Part model, mm, in its own coordinate system. A direction names the side the tool comes from. Round coordinates to 2 decimals unless told otherwise and drop trailing zeros. Write each loop counter-clockwise with the first axis right and the second up, starting at its lowest first coordinate (ties: lowest second). Pieces come first, ordered by that corner, then holes. Notation, with made-up numbers: M -27.75,-1 L 0.25,-1 A15 cw 0.25,18 Z; hole C 18,75.5 d5. An arc over 180 degrees is marked long. Answer as a JSON object with one key per item and string values. Group by question number.
1. Drop flat-ended pins along their axis: pin 1 (5.5 mm diameter, centred on x = 114.8, y = 74.5, fed in from +Z); pin 2 (1.6 mm diameter, centred on x = 92.5, z = 2, fed in from -Y); pin 3 (1 mm diameter, centred on x = 128.5, z = 1, fed in from -Y); pin 4 (1.6 mm diameter, centred on y = 8, z = 1.5, fed in from +X). Give the stop position or say it passes through.
2. Drill centre lines: line 1 (X direction, y = 74.5, z = 1); line 2 (Y direction, x = 114.8, z = 0.9); line 3 (X direction, y = 73, z = 2). Where is each one in solid material? Low to high. Write a range as from..to.
3. Band-saw the part on A-A, the plane y = 74.5. Write the cut outline in (x, z), plus the area to 3 significant figures.
4. Which spindle directions (+Z, -Z, +X, -X, +Y, -Y) get a long thin tool onto all of the face, cutting with end or side? Do faces 4 (the face through (2, 66.567, 2)), 5 (the face through (126.8, 8, 2)), 6 (the face through (72.322, 2, 2)), 7 (the face through (2, 13.233, 2)), 8 (the face through (128, 40.1, 2)). Say none if no direction does.
5. Band-saw the part on B-B, the plane z = 1.6. Count the separate pieces of the cut face and the enclosed holes in it, plus the area to 3 significant figures.
6. Band-saw the part on C-C, the plane y = 62.5. Write the cut outline in (x, z), plus the area to 3 significant figures.
7. Two-plate mould, pull along X, no slides. Class faces 1 (the face through (16, 73, 2)), 2 (the face through (130, 47, 2)), 3 (the face through (108, 0, 2)): +X half, -X half, draft (parallel to the pull), parting line (faces both ways), or undercut.
from build123d import *

# Parameters (mm, degrees)
SKETCH1_W           = 130
SKETCH1_H           = 80
BOSS_EXTRUDE1_DEPTH = 3.2
SKETCH2_W           = 14.444444444
SKETCH2_H           = 3.2
SKETCH2_W_2         = 3.2
SKETCH2_H_2         = 13.333333334
SKETCH2_H_3         = 13.333333333
CUT_EXTRUDE1_DEPTH  = 153.676913775
MOVE_FACE1_BY       = 0.1
MOVE_FACE1_2_BY     = 0.1
MOVE_FACE1_3_BY     = 0.1
MOVE_FACE1_4_BY     = 0.1
MOVE_FACE1_5_BY     = 0.1
MOVE_FACE1_6_BY     = 0.1
MOVE_FACE1_7_BY     = 0.1
MOVE_FACE1_8_BY     = 0.1
MOVE_FACE1_9_BY     = 0.1
MOVE_FACE1_10_BY    = 0.1
MOVE_FACE1_11_BY    = 0.1
MOVE_FACE1_12_BY    = 0.1
MOVE_FACE1_13_BY    = 0.1
MOVE_FACE1_14_BY    = 0.1
MOVE_FACE1_15_BY    = 0.1
MOVE_FACE1_16_BY    = 0.1
MOVE_FACE1_17_BY    = 0.1
MOVE_FACE1_18_BY    = 0.1
CUT_EXTRUDE2_REACH  = 154.677
SKETCH3_R           = 1.7
CUT_EXTRUDE3_REACH  = 154.677
SKETCH4_R           = 1.5


with BuildPart() as part:
    # Sketch1 → Boss-Extrude1 (new body)
    with BuildSketch(Plane.XY):
        with Locations((65, 40)):
            Rectangle(SKETCH1_W, SKETCH1_H)
    extrude(amount=BOSS_EXTRUDE1_DEPTH)

    # Sketch2 → Cut-Extrude1 (cut, through all)
    with BuildSketch(Plane.XY.offset(3.2)):
        with Locations((7.222222222, 1.6)):
            Rectangle(SKETCH2_W, SKETCH2_H)
        with Locations((36.111111111, 1.6)):
            Rectangle(SKETCH2_W, SKETCH2_H)
        with Locations((65, 1.6)):
            Rectangle(SKETCH2_W, SKETCH2_H)
        with Locations((93.888888889, 1.6)):
            Rectangle(SKETCH2_W, SKETCH2_H)
        Polygon((115.555555556, 0), (115.555555556, 3.2), (126.8, 3.2), (126.8, 13.333333333), (130, 13.333333333), (130, 0), align=None)
        with Locations((1.6, 20)):
            Rectangle(SKETCH2_W_2, SKETCH2_H_2)
        with Locations((1.6, 46.666666667)):
            Rectangle(SKETCH2_W_2, SKETCH2_H_3)
        with Locations((1.6, 73.333333334)):
            Rectangle(SKETCH2_W_2, SKETCH2_H_3)
        with Locations((128.4, 33.333333334)):
            Rectangle(SKETCH2_W_2, SKETCH2_H_3)
        with Locations((128.4, 60)):
            Rectangle(SKETCH2_W_2, SKETCH2_H_2)
    extrude(amount=-CUT_EXTRUDE1_DEPTH, mode=Mode.SUBTRACT)

    # Move Face1: a face moved inward by 0.1
    extrude(part.faces().sort_by_distance((128.4, 53.333333333, 1.6))[0], amount=MOVE_FACE1_BY, dir=(0, -1, 0), mode=Mode.SUBTRACT)

    # Move Face1 2: a face moved inward by 0.1
    extrude(part.faces().sort_by_distance((128.4, 26.666666667, 1.6))[0], amount=MOVE_FACE1_2_BY, dir=(0, -1, 0), mode=Mode.SUBTRACT)

    # Move Face1 3: a face moved inward by 0.1
    extrude(part.faces().sort_by_distance((128.4, 13.333333333, 1.6))[0], amount=MOVE_FACE1_3_BY, dir=(0, 1, 0), mode=Mode.SUBTRACT)

    # Move Face1 4: a face moved inward by 0.1
    extrude(part.faces().sort_by_distance((128.4, 40, 1.6))[0], amount=MOVE_FACE1_4_BY, dir=(0, 1, 0), mode=Mode.SUBTRACT)

    # Move Face1 5: a face moved inward by 0.1
    extrude(part.faces().sort_by_distance((128.4, 66.666666667, 1.6))[0], amount=MOVE_FACE1_5_BY, dir=(0, 1, 0), mode=Mode.SUBTRACT)

    # Move Face1 6: a face moved inward by 0.1
    extrude(part.faces().sort_by_distance((115.555555556, 1.6, 1.6))[0], amount=MOVE_FACE1_6_BY, dir=(-1, 0, 0), mode=Mode.SUBTRACT)

    # Move Face1 7: a face moved inward by 0.1
    extrude(part.faces().sort_by_distance((86.666666667, 1.6, 1.6))[0], amount=MOVE_FACE1_7_BY, dir=(-1, 0, 0), mode=Mode.SUBTRACT)

    # Move Face1 8: a face moved inward by 0.1
    extrude(part.faces().sort_by_distance((57.777777778, 1.6, 1.6))[0], amount=MOVE_FACE1_8_BY, dir=(-1, 0, 0), mode=Mode.SUBTRACT)

    # Move Face1 9: a face moved inward by 0.1
    extrude(part.faces().sort_by_distance((28.888888889, 1.6, 1.6))[0], amount=MOVE_FACE1_9_BY, dir=(-1, 0, 0), mode=Mode.SUBTRACT)

    # Move Face1 10: a face moved inward by 0.1
    extrude(part.faces().sort_by_distance((14.444444444, 1.6, 1.6))[0], amount=MOVE_FACE1_10_BY, dir=(1, 0, 0), mode=Mode.SUBTRACT)

    # Move Face1 11: a face moved inward by 0.1
    extrude(part.faces().sort_by_distance((43.333333333, 1.6, 1.6))[0], amount=MOVE_FACE1_11_BY, dir=(1, 0, 0), mode=Mode.SUBTRACT)

    # Move Face1 12: a face moved inward by 0.1
    extrude(part.faces().sort_by_distance((72.222222222, 1.6, 1.6))[0], amount=MOVE_FACE1_12_BY, dir=(1, 0, 0), mode=Mode.SUBTRACT)

    # Move Face1 13: a face moved inward by 0.1
    extrude(part.faces().sort_by_distance((101.111111111, 1.6, 1.6))[0], amount=MOVE_FACE1_13_BY, dir=(1, 0, 0), mode=Mode.SUBTRACT)

    # Move Face1 14: a face moved inward by 0.1
    extrude(part.faces().sort_by_distance((1.6, 26.666666667, 1.6))[0], amount=MOVE_FACE1_14_BY, dir=(0, 1, 0), mode=Mode.SUBTRACT)

    # Move Face1 15: a face moved inward by 0.1
    extrude(part.faces().sort_by_distance((1.6, 13.333333333, 1.6))[0], amount=MOVE_FACE1_15_BY, dir=(0, -1, 0), mode=Mode.SUBTRACT)

    # Move Face1 16: a face moved inward by 0.1
    extrude(part.faces().sort_by_distance((1.6, 40, 1.6))[0], amount=MOVE_FACE1_16_BY, dir=(0, -1, 0), mode=Mode.SUBTRACT)

    # Move Face1 17: a face moved inward by 0.1
    extrude(part.faces().sort_by_distance((1.6, 53.333333333, 1.6))[0], amount=MOVE_FACE1_17_BY, dir=(0, 1, 0), mode=Mode.SUBTRACT)

    # Move Face1 18: a face moved inward by 0.1
    extrude(part.faces().sort_by_distance((1.6, 66.666666667, 1.6))[0], amount=MOVE_FACE1_18_BY, dir=(0, -1, 0), mode=Mode.SUBTRACT)

    # Sketch3 → Cut-Extrude2 (cut, up to next)
    with BuildSketch(Plane.XY.offset(3.2), mode=Mode.PRIVATE) as cut_extrude2_sk1:
        with Locations((15.2, 74.5)):
            Circle(SKETCH3_R)
    cut_extrude2_tool1 = extrude(cut_extrude2_sk1.sketch, amount=-CUT_EXTRUDE2_REACH, mode=Mode.PRIVATE) & part.part
    # Sketch3 → Cut-Extrude2 (cut, up to next)
    with BuildSketch(Plane.XY.offset(3.2), mode=Mode.PRIVATE) as cut_extrude2_sk2:
        with Locations(Location((114.8, 74.5, 0), (0, 0, 180))):
            Circle(SKETCH3_R)
    cut_extrude2_tool2 = extrude(cut_extrude2_sk2.sketch, amount=-CUT_EXTRUDE2_REACH, mode=Mode.PRIVATE) & part.part
    add(cut_extrude2_tool1.solids().sort_by_distance((15.2, 74.5, 3.2))[0], mode=Mode.SUBTRACT)
    add(cut_extrude2_tool2.solids().sort_by_distance((114.8, 74.5, 3.2))[0], mode=Mode.SUBTRACT)

    # Sketch4 → Cut-Extrude3 (cut, up to next)
    with BuildSketch(Plane(origin=(0, 0, 0), x_dir=(-1, 0, 0), z_dir=(0, 0, -1)), mode=Mode.PRIVATE) as cut_extrude3_sk1:
        with Locations((-71.91, 16.56)):
            Circle(SKETCH4_R)
    cut_extrude3_tool1 = extrude(cut_extrude3_sk1.sketch, amount=-CUT_EXTRUDE3_REACH, mode=Mode.PRIVATE) & part.part
    add(cut_extrude3_tool1.solids().sort_by_distance((71.91, 16.56, 0))[0], mode=Mode.SUBTRACT)


solid = part.part
Worked answers:
{
 "1": {"pin 1": "stops at z = 3.2", "pin 2": "stops at y = 3.2", "pin 3": "stops at y = 13.43", "pin 4": "stops at x = 126.8"},
 "2": {"line 1": "x = 3.2..13.5, 16.9..113.1, 116.5..130", "line 2": "y = 0..72.8, 76.2..80", "line 3": "x = 3.2..14.4, 16..114, 115.6..130"},
 "3": {"outline": "M 3.2,0 L 13.5,0 L 13.5,3.2 L 3.2,3.2 Z; M 16.9,0 L 113.1,0 L 113.1,3.2 L 16.9,3.2 Z; M 116.5,0 L 130,0 L 130,3.2 L 116.5,3.2 Z", "area": "384 mm^2"},
 "4": {"face 4": "+Z, -Z, -X, +Y", "face 5": "+Z, -Z, +X, -Y", "face 6": "+Z, -Z, -Y", "face 7": "+Z, -Z, -X", "face 8": "+Z, -Z, +X"},
 "5": {"separate pieces": "1", "enclosed holes": "3", "area": "9,890 mm^2"},
 "6": {"outline": "M 0,0 L 126.8,0 L 126.8,3.2 L 0,3.2 Z", "area": "406 mm^2"},
 "7": {"face 1": "undercut", "face 2": "+X half", "face 3": "draft"}
}
